from build123d import *

# Parameters (mm, degrees)
F1_DEPTH  = 5.08
F3_DEPTH  = 101.6
F5_DEPTH  = 76.2
F7_DEPTH  = 127
F9_DEPTH  = 63.5
F11_DEPTH = 3.175
F12_R     = 1.27
F14_DEPTH = 25.4


with BuildPart() as f1:
    # F0 (on Top) → F1 (new body)
    with BuildSketch(Plane.XY):
        with BuildLine():
            Line((158.75, 0), (19.05, 0))
            ThreePointArc((19.05, 0), (5.5796158184, -5.5796158184), (0, -19.05))
            Line((0, -19.05), (0, -107.95))
            ThreePointArc((0, -107.95), (5.5796158184, -121.4203841816), (19.05, -127))
            Line((19.05, -127), (158.75, -127))
            ThreePointArc((158.75, -127), (172.2203841816, -121.4203841816), (177.8, -107.95))
            Line((177.8, -107.95), (177.8, -19.05))
            ThreePointArc((177.8, -19.05), (172.2203841816, -5.5796158184), (158.75, 0))
        make_face()
    extrude(amount=F1_DEPTH)

    # F2 (on face) → F3 (join)
    with BuildSketch(Plane.XY.offset(5.08)):
        with BuildLine():
            Line((57.6015881181, 0), (19.05, 0))
            ThreePointArc((19.05, 0), (5.5796158184, -5.5796158184), (0, -19.05))
            Line((0, -19.05), (0, -63.5))
            Line((0, -63.5), (57.6015881181, -63.5))
            Line((57.6015881181, -63.5), (57.6015881181, 0))
        make_face()
        with BuildLine():
            ThreePointArc((3.175, -22.225), (8.7546158184, -8.7546158184), (22.225, -3.175))
            Line((22.225, -3.175), (54.4265881181, -3.175))
            Line((54.4265881181, -3.175), (54.4265881181, -60.325))
            Line((54.4265881181, -60.325), (3.175, -60.325))
            Line((3.175, -60.325), (3.175, -22.225))
        make_face(mode=Mode.SUBTRACT)
    extrude(amount=F3_DEPTH)

    # F4 (on face) → F5 (join)
    with BuildSketch(Plane.XY.offset(5.08)):
        with BuildLine():
            Line((3.175, -63.5), (0, -63.5))
            Line((0, -63.5), (0, -107.95))
            ThreePointArc((0, -107.95), (5.5796158184, -121.4203841816), (19.05, -127))
            Line((19.05, -127), (57.6015881181, -127))
            Line((57.6015881181, -127), (57.6015881181, -63.5))
            Line((57.6015881181, -63.5), (54.4265881181, -63.5))
            Line((54.4265881181, -63.5), (54.4265881181, -123.825))
            Line((54.4265881181, -123.825), (22.225, -123.825))
            ThreePointArc((22.225, -123.825), (8.7546158184, -118.2453841816), (3.175, -104.775))
            Line((3.175, -104.775), (3.175, -63.5))
        make_face()
    extrude(amount=F5_DEPTH)

    # F6 (on face) → F7 (join)
    with BuildSketch(Plane.XY.offset(5.08)):
        with BuildLine():
            Line((54.4265881181, 0), (54.4265881181, -63.5))
            Line((54.4265881181, -63.5), (111.5765881181, -63.5))
            Line((111.5765881181, -63.5), (111.5765881181, -19.05))
            ThreePointArc((111.5765881181, -19.05), (105.9969722997, -5.5796158184), (92.5265881181, 0))
            Line((92.5265881181, 0), (57.6015881181, 0))
            Line((57.6015881181, 0), (54.4265881181, 0))
        make_face()
        with BuildLine():
            Line((57.6015881181, -60.325), (57.6015881181, -3.175))
            Line((57.6015881181, -3.175), (89.3515881181, -3.175))
            ThreePointArc((89.3515881181, -3.175), (102.8219722997, -8.7546158184), (108.4015881181, -22.225))
            Line((108.4015881181, -22.225), (108.4015881181, -60.325))
            Line((108.4015881181, -60.325), (57.6015881181, -60.325))
        make_face(mode=Mode.SUBTRACT)
    extrude(amount=F7_DEPTH)

    # F8 (on face) → F9 (join)
    with BuildSketch(Plane.XY.offset(5.08)):
        with BuildLine():
            Line((111.5765881181, -60.325), (54.4265881181, -60.325))
            Line((54.4265881181, -60.325), (54.4265881181, -127))
            Line((54.4265881181, -127), (92.5265881181, -127))
            ThreePointArc((92.5265881181, -127), (105.9969722997, -121.4203841816), (111.5765881181, -107.95))
            Line((111.5765881181, -107.95), (111.5765881181, -60.325))
        make_face()
        with BuildLine():
            Line((57.6015881181, -123.825), (57.6015881181, -63.5))
            Line((57.6015881181, -63.5), (108.4015881181, -63.5))
            Line((108.4015881181, -63.5), (108.4015881181, -104.775))
            ThreePointArc((108.4015881181, -104.775), (102.8219722997, -118.2453841816), (89.3515881181, -123.825))
            Line((89.3515881181, -123.825), (57.6015881181, -123.825))
        make_face(mode=Mode.SUBTRACT)
    extrude(amount=F9_DEPTH)

    # F10 (on face) → F11 (join)
    with BuildSketch(Plane.XY.offset(5.08)):
        with BuildLine():
            Line((158.75, 0), (92.5265881181, 0))
            Line((92.5265881181, 0), (103.0568718275, -3.175))
            Line((103.0568718275, -3.175), (155.575, -3.175))
            ThreePointArc((155.575, -3.175), (169.0453841816, -8.7546158184), (174.625, -22.225))
            Line((174.625, -22.225), (174.625, -104.775))
            ThreePointArc((174.625, -104.775), (169.0453841816, -118.2453841816), (155.575, -123.825))
            Line((155.575, -123.825), (103.0568718275, -123.825))
            Line((103.0568718275, -123.825), (92.5265881181, -127))
            Line((92.5265881181, -127), (158.75, -127))
            ThreePointArc((158.75, -127), (172.2203841816, -121.4203841816), (177.8, -107.95))
            Line((177.8, -107.95), (177.8, -19.05))
            ThreePointArc((177.8, -19.05), (172.2203841816, -5.5796158184), (158.75, 0))
        make_face()
    extrude(amount=F11_DEPTH)

    # F12
    f12_edges = [f1.edges().sort_by_distance(p)[0] for p in [
        (125.638294, 0, 8.255),
        (169.045384, -8.754616, 8.255),
        (172.220384, -5.579616, 8.255),
        (177.8, -63.5, 8.255),
        (174.625, -63.5, 8.255),
        (172.220384, -121.420384, 8.255),
        (169.045384, -118.245384, 8.255),
        (129.315936, -123.825, 8.255),
        (125.638294, -127, 8.255),
        (129.315936, -3.175, 8.255),
    ]]
    fillet(f12_edges, radius=F12_R)

    # F13 (on face) → F14 (join)
    with BuildSketch(Plane.XY.offset(5.08)):
        with BuildLine():
            Line((111.5765881181, -92.075), (127.4515881181, -92.075))
            ThreePointArc((127.4515881181, -92.075), (136.4318442391, -88.3552561211), (140.1515881181, -79.375))
            Line((140.1515881181, -79.375), (140.1515881181, -47.625))
            ThreePointArc((140.1515881181, -47.625), (136.4318442391, -38.6447438789), (127.4515881181, -34.925))
            Line((127.4515881181, -34.925), (111.5765881181, -34.925))
            Line((111.5765881181, -34.925), (111.5765881181, -38.1))
            Line((111.5765881181, -38.1), (124.2765881181, -38.1))
            ThreePointArc((124.2765881181, -38.1), (133.2568442391, -41.8197438789), (136.9765881181, -50.8))
            Line((136.9765881181, -50.8), (136.9765881181, -76.2))
            ThreePointArc((136.9765881181, -76.2), (133.2568442391, -85.1802561211), (124.2765881181, -88.9))
            Line((124.2765881181, -88.9), (111.5765881181, -88.9))
            Line((111.5765881181, -88.9), (111.5765881181, -92.075))
        make_face()
    extrude(amount=F14_DEPTH)


solid = f1.part
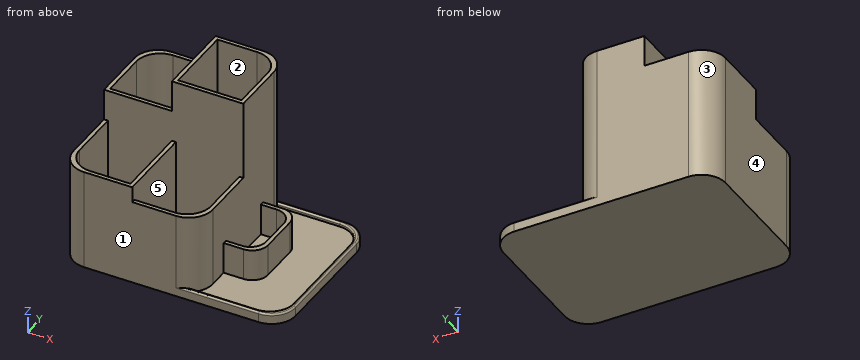
Design review of the part built by this model. Coordinates are the model's own, in mm. Face numbers are marked on the shaded views. A direction names the side the tool comes from. Give positions to 0.01 mm unless a question says otherwise; leave off trailing zeros. Loops run counter-clockwise (first coordinate to the right, second up) from the corner with the lowest first, then second, coordinate; pieces in that order, holes last. Notation, with made-up numbers: (0.5, -25) - (27.5, -25) arc R19 cw to (27.5, -21) - close; hole circle Ø5 at (-31.75, 88). An arc over 180 degrees is marked (long way). Write item = value, one per line.
1) Take a section at B-B on y = -25. State the section outline as (x, z) points (3 decimals), and give its area (3 significant figures).
Result sheet:
outline = (0, 0) - (177.8, 0) - (177.8, 6.985) arc R1.27 ccw to (176.53, 8.255) - (175.895, 8.255) arc R1.27 ccw to (174.625, 6.985) - (174.625, 5.08) - (111.577, 5.08) - (111.577, 132.08) - (108.402, 132.08) - (108.402, 5.08) - (57.602, 5.08) - (57.602, 132.08) - (54.427, 132.08) - (54.427, 5.08) - (3.175, 5.08) - (3.175, 106.68) - (0, 106.68) - close
area = 2,040 mm2
2) Tool access review of the marked faces 4 and 5: name each direction out of +Z, -Z, +X, -X, +Y, -Y from which nothing blocks a thin tool from reaching the whole face with its end or side.
Result sheet:
face_4 = +Z, -Z, -X, +Y, -Y
face_5 = +Z
3) Take a section at A-A on z = 100. State the section outline as (x, y) points (3 decimals).
Result sheet:
outline = (0, -63.5) - (111.577, -63.5) - (111.577, -19.05) arc R19.05 ccw to (92.527, 0) - (19.05, 0) arc R19.05 ccw to (0, -19.05) - close; hole (3.175, -60.325) - (54.427, -60.325) - (54.427, -3.175) - (22.225, -3.175) arc R19.05 ccw to (3.175, -22.225) - close; hole (57.602, -60.325) - (108.402, -60.325) - (108.402, -22.225) arc R19.05 ccw to (89.352, -3.175) - (57.602, -3.175) - close
4) Take a section at D-D on x = 42. State the section outline as (y, z) points (3 decimals), and give its area (3 significant figures).
Result sheet:
outline = (-127, 0) - (0, 0) - (0, 106.68) - (-3.175, 106.68) - (-3.175, 5.08) - (-60.325, 5.08) - (-60.325, 106.68) - (-63.5, 106.68) - (-63.5, 5.08) - (-123.825, 5.08) - (-123.825, 81.28) - (-127, 81.28) - close
area = 1,530 mm2
5) Clearance check with flat-ended pins moving along their axes: pin 1 Ø1.5 at (x, y) = (55, -89.5) entering from +Z; pin 2 Ø6.5 at (x, z) = (120, 23.5) entering from +Y (3 decimals); pin 3 Ø15.5 at (x, y) = (17.5, -95.5) entering from +Z. State where each tip first meets the part, or that it passes through.
Result sheet:
pin_1 = 81.28
pin_2 = -34.925
pin_3 = 5.08
6) To check wall thickness, follow line 1 (Y direction, x = 68, z = 24.5) (3 decimals); line 2 (X direction, y = -42, z = 71) (3 decimals); line 3 (X direction, y = -61.5, z = 7). State the ranges of each line that lie inside material, in increasing order.
Result sheet:
line_1 = -127 to -123.825, -63.5 to -60.325, -3.175 to 0
line_2 = 0 to 3.175, 54.427 to 57.602, 108.402 to 111.577
line_3 = 0 to 111.58, 136.98 to 140.15, 174.63 to 177.8
7) Draft analysis for pull direction X (two halves, no side actions). For the marked faces 1, 2 and 3, state which applies: +X half, -X half, draft (parallel to the pull), parting line (faces both ways), or undercut.
Result sheet:
face_1 = draft
face_2 = undercut
face_3 = -X half
8) Take a section at C-C on z = 56. State the section outline as (x, y) points (3 decimals), and give its area (3 significant figures).
Result sheet:
outline = (0, -107.95) arc R19.05 ccw to (19.05, -127) - (92.527, -127) arc R19.05 ccw to (111.577, -107.95) - (111.577, -19.05) arc R19.05 ccw to (92.527, 0) - (19.05, 0) arc R19.05 ccw to (0, -19.05) - close; hole (3.175, -104.775) arc R19.05 ccw to (22.225, -123.825) - (54.427, -123.825) - (54.427, -63.5) - (3.175, -63.5) - close; hole (3.175, -60.325) - (54.427, -60.325) - (54.427, -3.175) - (22.225, -3.175) arc R19.05 ccw to (3.175, -22.225) - close; hole (57.602, -123.825) - (89.352, -123.825) arc R19.05 ccw to (108.402, -104.775) - (108.402, -63.5) - (57.602, -63.5) - close; hole (57.602, -60.325) - (108.402, -60.325) - (108.402, -22.225) arc R19.05 ccw to (89.352, -3.175) - (57.602, -3.175) - close
area = 2,180 mm2
